Can you work these out from the model? Positions are in its coordinate system, mm. A direction names the side the tool comes from. Give positions to 0.01 mm unless a question says otherwise; leave off trailing zeros. Order: outer loops, then holes, each group sorted by start corner. A loop starts at its lowest first (then second) coordinate and runs counter-clockwise, first axis right, second up. Notation, with made-up numbers: M 71.5,65.25 L 93.5,65.25 A28 cw 93.5,83.25 Z; hole C -39.5,-30.5 d3. An arc over 180 degrees is marked long. Answer as a JSON object with one key per item and string values.
```python
from build123d import *

# Parameters (mm, degrees)
SKETCH1_R           = 27
SKETCH1_R_2         = 22.5
BOSS_EXTRUDE1_DEPTH = 10
SKETCH2_R           = 1.6
CUT_EXTRUDE1_DEPTH  = 11


with BuildPart() as part:
    # Sketch1 → Boss-Extrude1 (new body)
    with BuildSketch(Plane.XY):
        with BuildLine():
            Line((-48.092977135, -207.645932851), (-123.092977135, -207.645932851))
            ThreePointArc((-123.092977135, -207.645932851), (-137.235112759, -201.788068475), (-143.092977135, -187.645932851))
            Line((-143.092977135, -187.645932851), (-143.092977135, -153.645932851))
            ThreePointArc((-143.092977135, -153.645932851), (-137.235112759, -139.503797227), (-123.092977135, -133.645932851))
            Line((-123.092977135, -133.645932851), (-48.092977135, -133.645932851))
            ThreePointArc((-48.092977135, -133.645932851), (-31.673163065, -137.488886754), (-18.664191619, -148.219462263))
            Line((-18.664191619, -148.219462263), (-14.592977135, -148.219462263))
            ThreePointArc((-14.592977135, -148.219462263), (-11.05744323, -149.683928357), (-9.592977135, -153.219462263))
            Line((-9.592977135, -153.219462263), (-9.592977135, -188.072403439))
            ThreePointArc((-9.592977135, -188.072403439), (-11.05744323, -191.607937345), (-14.592977135, -193.072403439))
            Line((-14.592977135, -193.072403439), (-18.664191619, -193.072403439))
            ThreePointArc((-18.664191619, -193.072403439), (-31.673163065, -203.802978948), (-48.092977135, -207.645932851))
        make_face()
        with Locations((-48.092977135, -170.645932851)):
            Circle(SKETCH1_R, mode=Mode.SUBTRACT)
        with Locations((-114.092977135, -170.645932851)):
            Circle(SKETCH1_R_2, mode=Mode.SUBTRACT)
    extrude(amount=-BOSS_EXTRUDE1_DEPTH)

    # Sketch2 → Cut-Extrude1 (cut, through all)
    with BuildSketch(Plane.XY):
        with Locations((-48.092977135, -202.395935058)):
            Circle(SKETCH2_R)
    extrude(amount=-CUT_EXTRUDE1_DEPTH, mode=Mode.SUBTRACT)


solid = part.part
```
1) I want a section at C-C on z = -8.5. Write out the boundary of the cut face in (x, y), and give its area (3 significant figures).
Results found:
{"outline": "M -143.09,-187.65 A20 ccw -123.09,-207.65 L -48.09,-207.65 A37 ccw -18.66,-193.07 L -14.59,-193.07 A5 ccw -9.59,-188.07 L -9.59,-153.22 A5 ccw -14.59,-148.22 L -18.66,-148.22 A37 ccw -48.09,-133.65 L -123.09,-133.65 A20 ccw -143.09,-153.65 Z; hole C -114.09,-170.65 d45; hole C -48.09,-170.65 d54; hole C -48.09,-202.4 d3.2", "area": "5,280 mm²"}
2) I'm going to push flat-ended pins straight in: pin 1 Ø3.5 at (x, z) = (-17, -5) entering from -Y; pin 2 Ø2 at (x, z) = (-17, -4) entering from +Y; pin 3 Ø8 at (x, y) = (-119, -153.5) entering from -Z; pin 4 Ø4 at (y, z) = (-191, -8) entering from -X. Where does each tip first touch, or does it pass through?
Results found:
{"pin 1": "stops at y = -193.18", "pin 2": "stops at y = -148.22", "pin 3": "passes through", "pin 4": "stops at x = -143.05"}
3) I need wall thicknesses on L1, parallel to X at y = -171, z = -4; L2, parallel to Y at x = -115, z = -2; L3, parallel to X at y = -162, z = -7. Which ranges of each line are inside material? Lowest first, please.
Results found:
{"L1": "x = -143.09 to -136.59, -91.6 to -75.09, -21.1 to -9.59", "L2": "y = -207.65 to -193.13, -148.16 to -133.65", "L3": "x = -143.09 to -134.87, -93.32 to -73.67, -22.51 to -9.59"}
4) Thinking about a two-plate mould opening in Y: for faces 4 (the face through (-137.08, -201.94, -4.93)), 5 (the face through (-69.5, -187.1, -4.9)), 6 (the face through (-143.093, -171, -5)), which applies, pulls with the +Y half, pulls with the -Y half, needs draft (parallel to the pull), parting line crosses it, or undercut?
Results found:
{"face 4": "pulls with the -Y half", "face 5": "undercut", "face 6": "needs draft"}
5) I want a section at D-D on x = -43. Write out the boundary of the cut face in (y, z).
Results found:
{"outline": "M -207.29,-10 L -197.16,-10 L -197.16,0 L -207.29,0 Z; M -144.13,-10 L -134,-10 L -134,0 L -144.13,0 Z"}
6) I want a section at B-B on y = -190. Write out the boundary of the cut face in (x, z), and give its area (3 significant figures).
Results found:
{"outline": "M -142.95,-10 L -125.57,-10 L -125.57,0 L -142.95,0 Z; M -102.62,-10 L -66.92,-10 L -66.92,0 L -102.62,0 Z; M -29.27,-10 L -9.98,-10 L -9.98,0 L -29.27,0 Z", "area": "724 mm²"}
7) For faces 1 (the face through (-137.39, -139.66, -4.93)), 2 (the face through (-17, -193.072, -5)), 3 (the face through (-17, -148.219, -5)), which set-ups out of +Z, -Z, +X, -X, +Y, -Y let a thin tool reach every point of the face, with its end or its side?
Results found:
{"face 1": "+Z, -Z, -X, +Y", "face 2": "+Z, -Z, +X, -Y", "face 3": "+Z, -Z, +X, +Y"}
8) I want a section at A-A on x = -135. Write out the boundary of the cut face in (y, z).
Results found:
{"outline": "M -203.72,-10 L -178.96,-10 L -178.96,0 L -203.72,0 Z; M -162.33,-10 L -137.58,-10 L -137.58,0 L -162.33,0 Z"}
